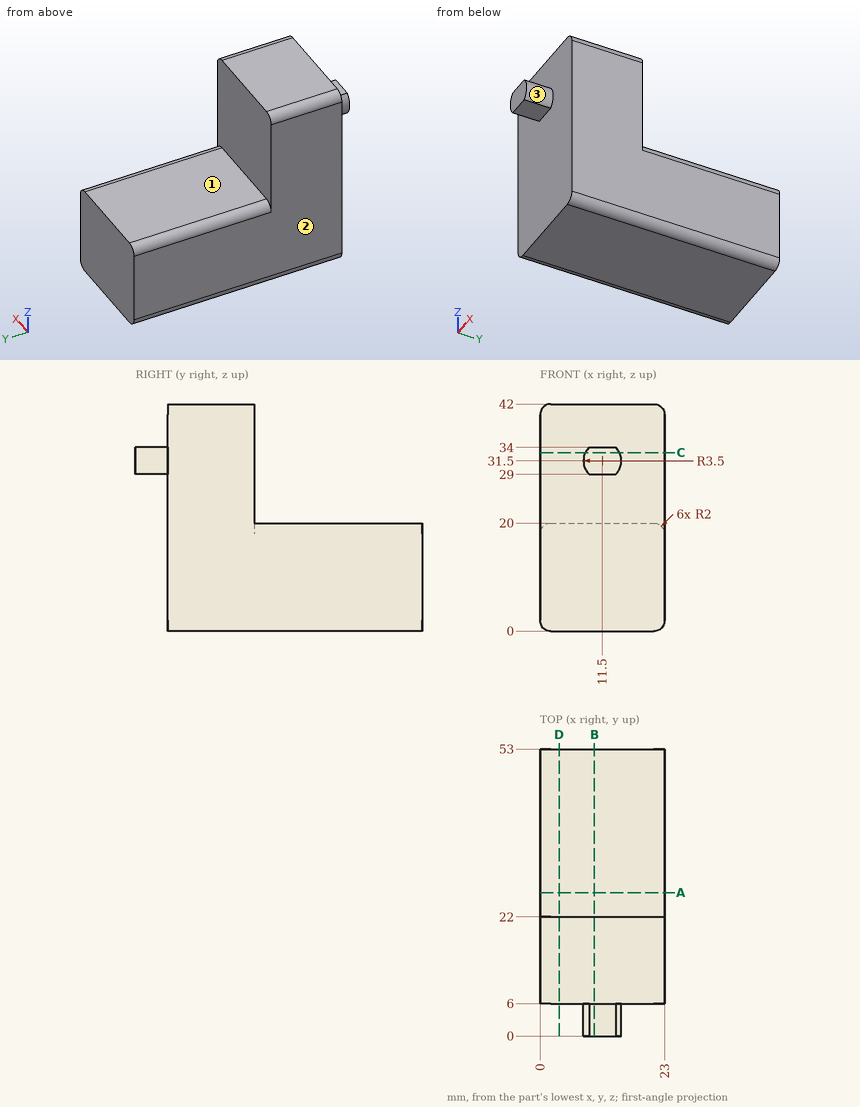
Part print with two shaded views. Sizes in mm from the minimum x, y, z corner. A direction names the side the tool comes from. Round coordinates to 2 decimals unless told otherwise and drop trailing zeros. Order: outer loops, then holes, each group sorted by start corner. A loop starts at its lowest first (then second) coordinate and runs counter-clockwise, first axis right, second up. Notation, with made-up numbers: (7.25, -39) -> (39.25, -39) arc R35 ccw to (39.25, -6) -> close; hole circle Ø11 at (53.25, -32.5). An arc over 180 degrees is marked (long way). Write each question's results on one line, items separated by ' | '.
1. Cut at B-B (x = 10). Give the cut face in (y, z), plus the area to 3 significant figures.
Findings below:
outline: (0, 29) -> (6, 29) -> (6, 0) -> (53, 0) -> (53, 20) -> (22, 20) -> (22, 42) -> (6, 42) -> (6, 34) -> (0, 34) -> close | area: 1,320 mm²
2. Cut at A-A (y = 26.5). Give the cut face in (x, z), plus the area to 3 significant figures.
Findings below:
outline: (0, 2) arc R2 ccw to (2, 0) -> (21, 0) arc R2 ccw to (23, 2) -> (23, 18) arc R2 ccw to (21, 20) -> (2, 20) arc R2 ccw to (0, 18) -> close | area: 457 mm²
3. Wall check: line 1 along Z through (x, y) = (17.25, 24.5); line 2 along Y through (x, z) = (4.25, 31); line 3 along Y through (x, z) = (2.75, 7.5). Give the ranges that are in metal, low to high. Write a range as [from, to].
Findings below:
line 1: z = [0, 20] | line 2: y = [6, 22] | line 3: y = [6, 53]
4. 3-axis set-ups, long thin cutter, end or side, ignore diameter. For the marked faces 1, 2 and 3: which of +Z, -Z, +X, -X, +Y, -Y reach the whole face in a straight line?
Findings below:
face 1: +Z, +X, -X, +Y | face 2: +Z, -Z, -X, +Y, -Y | face 3: +X, -Y
5. Cut at D-D (x = 3.5). Give the cut face in (y, z).
Findings below:
outline: (6, 0) -> (53, 0) -> (53, 20) -> (22, 20) -> (22, 42) -> (6, 42) -> close
6. Flat gauge pins, fed straight in: P1, Ø1.5, axis at x = 12, y = 3, coming from the +Z side; P2, Ø8, axis at x = 20, z = 13, coming from the -Y side; P3, Ø5.5, axis at x = 11.5, y = 32.5, coming from the +Z side. Where does each tip first touch, or does it go through?
Findings below:
P1: stops at z = 34 | P2: stops at y = 6 | P3: stops at z = 20
7. Cut at C-C (z = 33). Give the cut face in (x, y), plus the area to 3 significant figures.
Findings below:
outline: (0, 6) -> (8.34, 6) -> (8.34, 0) -> (14.66, 0) -> (14.66, 6) -> (23, 6) -> (23, 22) -> (0, 22) -> close | area: 406 mm²
